from build123d import *

# Parameters (mm, degrees)
F0_W     = 90
F0_H     = 41.77
F1_DEPTH = 6
F3_DEPTH = 28.33
F4_R     = 3
F5_R     = 1.5
F6_DEPTH = 5


with BuildPart() as f1:
    # F0 (on Front) → F1 (new body, symmetric)
    with BuildSketch(Plane.XZ):
        Rectangle(F0_W, F0_H)
    extrude(amount=F1_DEPTH, both=True)

    # F2 (on face) → F3 (join)
    with BuildSketch(Plane.XY.offset(20.885)):
        with BuildLine():
            Line((-28, 0), (-23, 0))
            ThreePointArc((-23, 0), (-28, 5), (-33, 0))
            Line((-33, 0), (-28, 0))
        make_face()
        with BuildLine():
            ThreePointArc((-33, 0), (-28, -5), (-23, 0))
            Line((-23, 0), (-28, 0))
            Line((-28, 0), (-33, 0))
        make_face()
        with BuildLine():
            Line((-5, 0), (0, 0))
            Line((0, 0), (5, 0))
            ThreePointArc((5, 0), (0, 5), (-5, 0))
        make_face()
        with BuildLine():
            Line((5, 0), (0, 0))
            Line((0, 0), (-5, 0))
            ThreePointArc((-5, 0), (0, -5), (5, 0))
        make_face()
        with BuildLine():
            ThreePointArc((33, 0), (28, 5), (23, 0))
            ThreePointArc((23, 0), (28, -5), (33, 0))
        make_face()
    extrude(amount=F3_DEPTH)

    # F4
    f4_edges = [f1.edges().sort_by_distance(p)[0] for p in [
        (45, -6, 0),
        (45, 6, 0),
        (-45, -6, 0),
        (-45, 6, 0),
    ]]
    fillet(f4_edges, radius=F4_R)

    # F5 (on face) → F6 (join)
    with BuildSketch(Plane.XY.offset(49.215)):
        with Locations((-28, 0)):
            Circle(F5_R)
        Circle(F5_R)
        with Locations((28, 0)):
            Circle(F5_R)
    extrude(amount=F6_DEPTH)


solid = f1.part
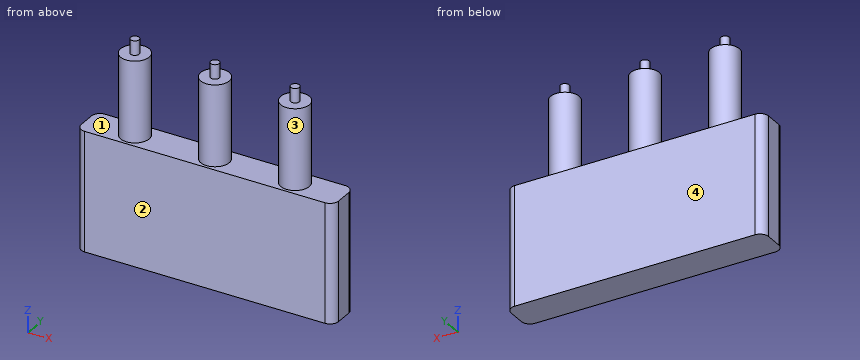
The model under review builds one solid part; all positions refer to its coordinate system, in mm. Face numbers are marked on the shaded views. A direction names the side the tool comes from. Coordinates: 2 decimals unless noted, no trailing zeros. Loops run counter-clockwise (first coordinate to the right, second up) from the corner with the lowest first, then second, coordinate; pieces in that order, holes last.
(1) Consider section B-B, the plane x = 0. Give the boundary of the cut face in (y, z) (3 decimals), plus the area to 3 significant figures.
Determined:
outline: (-6, -20.885) - (6, -20.885) - (6, 20.885) - (5, 20.885) - (5, 49.215) - (1.5, 49.215) - (1.5, 54.215) - (-1.5, 54.215) - (-1.5, 49.215) - (-5, 49.215) - (-5, 20.885) - (-6, 20.885) - close
area: 800 mm2
(2) Tool access review of the marked faces 3 and 4: name each direction out of +Z, -Z, +X, -X, +Y, -Y from which nothing blocks a thin tool from reaching the whole face with its end or side.
Determined:
face 3: +Z
face 4: +Z, -Z, +X, -X, +Y
(3) Draft analysis for pull direction X (two halves, no side actions). For the marked faces 1 and 2, state which applies: +X half, -X half, draft (parallel to the pull), parting line (faces both ways), or undercut.
Determined:
face 1: undercut
face 2: draft
(4) Consider section D-D, the plane x = 9.5. Give the boundary of the cut face in (y, z) (3 decimals).
Determined:
outline: (-6, -20.885) - (6, -20.885) - (6, 20.885) - (-6, 20.885) - close
(5) Consider section A-A, the plane y = 0. Give the boundary of the cut face in (x, z) (3 decimals), plus the area to 3 significant figures.
Determined:
outline: (-45, -20.885) - (45, -20.885) - (45, 20.885) - (33, 20.885) - (33, 49.215) - (29.5, 49.215) - (29.5, 54.215) - (26.5, 54.215) - (26.5, 49.215) - (23, 49.215) - (23, 20.885) - (5, 20.885) - (5, 49.215) - (1.5, 49.215) - (1.5, 54.215) - (-1.5, 54.215) - (-1.5, 49.215) - (-5, 49.215) - (-5, 20.885) - (-23, 20.885) - (-23, 49.215) - (-26.5, 49.215) - (-26.5, 54.215) - (-29.5, 54.215) - (-29.5, 49.215) - (-33, 49.215) - (-33, 20.885) - (-45, 20.885) - close
area: 4,650 mm2
(6) Insertion check: P1, Ø2, axis at y = 4, z = 25, coming from the +X side; P2, Ø1.5, axis at x = -8.5, y = -4.5, coming from the +Z side (3 decimals). Each pin has a flat end and moves straight along its axis. Give the tip position at first contact, or say it passes through.
Determined:
P1: stops at x = 32
P2: stops at z = 20.885
(7) Wall thickness on L1, parallel to X at y = -4.5, z = 44; L2, parallel to X at y = -2.75, z = 38.5; L3, parallel to Z at x = 36, y = 3.75 (3 decimals): over which ranges is each line inside the solid? List them lowest first.
Determined:
L1: x = -30.18 to -25.82, -2.18 to 2.18, 25.82 to 30.18
L2: x = -32.18 to -23.82, -4.18 to 4.18, 23.82 to 32.18
L3: z = -20.885 to 20.885
(8) Consider section C-C, the plane z = 43. Give the boundary of the cut face in (x, y), plus the area to 3 significant figures.
Determined:
outline: circle Ø10 at (-28, 0); circle Ø10 at (0, 0); circle Ø10 at (28, 0)
area: 236 mm2
